Read the model definition and answer for the solid it produces. Units are mm, in the model's axes. A direction names the side the tool comes from. Coordinates: 2 decimals unless noted, no trailing zeros. Write each loop counter-clockwise with the first axis right and the second up, starting at its lowest first coordinate (ties: lowest second). Pieces come first, ordered by that corner, then holes.
(1) Section A-A on z = 1425 is taken. Write down the section's boundary in (x, y).
(2) Section B-B on x = -10 is taken. Write down the section's boundary in (y, z), then the cut area to 3 significant figures.
(3) Find the intervals of material crossed by probe 1 along X at (y, z) = (-5, 918); probe 2 along X at (y, z) = (31.5, 177.5); probe 3 along Y at (x, z) = (77.5, 805.5), in increasing order.
(4) Which of the six approach directions +Z, -Z, +X, -X, +Y, -Y give full straight-line access (tool end or side, diameter ignored) to faces 4 (the cylindrical face through (-16.509, -25.07, 474.575)), 5 (the flat face through (180, 36, 912))?
(5) Given pin 1 (8 mm diameter, centred on x = -105.5, z = 644, fed in from +Y); pin 2 (6 mm diameter, centred on y = 36, z = 527, fed in from -X); pin 3 (1 mm diameter, centred on x = -21, z = 1068, fed in from +Y), each flat-ended and moving along its own axis, determine where each tip first touches the part or whether it passes through.
(6) Section C-C on y = 48 is taken. Write down the section's boundary in (x, z).
(7) Section D-D on z = 348 is taken. Write down the section's boundary in (x, y).
(8) The mould has two halves that part along X. Classify faces 1 (the cylindrical face through (13.07, -25.07, 1380.64)), 2 (the flat face through (70.49, -23.61, 1736.02)), 3 (the flat face through (190, 29, 912)): +X half, -X half, draft (parallel to the pull), parting line (faces both ways), or undercut.
from build123d import *

# Parameters (mm, degrees)
F1_DEPTH = 1850
F3_DEPTH = 200
F4_R     = 50
F5_DEPTH = 120.001


# Not quite as in the source:
# - a feature names something its author has since deleted; it is built from what else it names


with BuildPart() as f1:
    # F0 (on Top) → F1 (new body)
    with BuildSketch(Plane.XY):
        Polygon((-100, 0), (-110, 0), (-110, -30), (190, -30), (190, 90), (180, 90), (180, -20), (-100, -20), align=None)
    extrude(amount=F1_DEPTH)

    # F2 (on face) → F3 (cut)
    with BuildSketch(Plane.XZ.offset(30)):
        Polygon((186.4785214056, 0), (-110, 291.3486315578), (-110, 0), align=None)
        Polygon((-110, 1850), (-110, 1558.6513684422), (186.4785214056, 1850), align=None)
    extrude(amount=-F3_DEPTH, mode=Mode.SUBTRACT)

    # F4 (on face) → F5 (cut, through all)
    with BuildSketch(Plane.XZ.offset(30)):
        with Locations((-10, 425)):
            Circle(F4_R)
        with Locations((-10, 1425)):
            Circle(F4_R)
    extrude(amount=-F5_DEPTH, mode=Mode.SUBTRACT)


solid = f1.part
Response:
1. outline: (-110, -30) - (-60, -30) - (-60, -20) - (-100, -20) - (-100, 0) - (-110, 0) - close; (40, -30) - (190, -30) - (190, 90) - (180, 90) - (180, -20) - (40, -20) - close
2. outline: (-30, 193.08) - (-20, 193.08) - (-20, 375) - (-30, 375) - close; (-30, 475) - (-20, 475) - (-20, 1375) - (-30, 1375) - close; (-30, 1475) - (-20, 1475) - (-20, 1656.92) - (-30, 1656.92) - close
2. area: 12,600 mm2
3. probe 1: x = -110 to -100, 180 to 190
3. probe 2: x = 180 to 190
3. probe 3: y = -30 to -20
4. face 4: +Y, -Y
4. face 5: +Z, -Z, +Y
5. pin 1: stops at y = 0
5. pin 2: stops at x = 180
5. pin 3: stops at y = -20
6. outline: (180, 6.37) - (186.48, 0) - (190, 0) - (190, 1850) - (186.48, 1850) - (180, 1843.63) - close
7. outline: (-110, -30) - (190, -30) - (190, 90) - (180, 90) - (180, -20) - (-100, -20) - (-100, 0) - (-110, 0) - close
8. face 1: undercut
8. face 2: -X half
8. face 3: +X half
